For this review, take the finished solid that the model builds, in its own axes (mm). A direction names the side the tool comes from. Coordinates: 2 decimals unless noted, no trailing zeros. Order: outer loops, then holes, each group sorted by start corner. A loop starts at its lowest first (then second) coordinate and runs counter-clockwise, first axis right, second up. Notation, with made-up numbers: M 0.5,78 L 54.5,78 A20 ccw 54.5,115 Z; hole C 39.25,-29.5 d8. An arc over 180 degrees is marked long. Use one line per item in the form item = value. Start each with the question number.
```python
from build123d import *

# Parameters (mm, degrees)
SKETCH_1_R               = 5.65
SKETCH_1_R_2             = 4.15
EXTRUDE_1_DEPTH          = 8
SKETCH_1_3_R             = 11
SKETCH_1_3_R_2           = 5.65
EXTRUDE_2_DEPTH          = 4.75
CUT_EXTRUDE_1_DEPTH      = 3.5
CUT_EXTRUDE_START        = -3.25
CUT_EXTRUDE_3_DEPTH      = 3.25
CUT_EXTRUDE_START_2      = -10
CUT_EXTRUDE_4_DEPTH      = 10
PATTERN_CIRCULAR_1_COUNT = 35


with BuildPart() as part:
    # 草图1 → 凸台-拉伸1 (new body)
    with BuildSketch(Plane(origin=(0, 0, 0), x_dir=(1, 0, 0), z_dir=(0, 1, 0))):
        with Locations(Location((0, 0, 0), (0, 0, 270))):
            Circle(SKETCH_1_R)
        with Locations(Location((0, 0, 0), (0, 0, 270))):
            Circle(SKETCH_1_R_2, mode=Mode.SUBTRACT)
    extrude(amount=EXTRUDE_1_DEPTH)

    # 草图1<3> → 凸台-拉伸2 (add)
    with BuildSketch(Plane(origin=(0, 0, 0), x_dir=(1, 0, 0), z_dir=(0, 1, 0))):
        with Locations(Location((0, 0, 0), (0, 0, 270))):
            Circle(SKETCH_1_3_R)
        with Locations(Location((0, 0, 0), (0, 0, 270))):
            Circle(SKETCH_1_3_R_2, mode=Mode.SUBTRACT)
    extrude(amount=EXTRUDE_2_DEPTH)

    # 草图2 → 切除-拉伸1 (cut)
    with BuildSketch(Plane.XZ):
        Polygon((0, -7.274613392), (-6.3, -3.637306696), (-6.3, 3.637306696), (0, 7.274613392), (6.3, 3.637306696), (6.3, -3.637306696), align=None)
    extrude(amount=-CUT_EXTRUDE_1_DEPTH, mode=Mode.SUBTRACT)

    # 草图4 → 切除-拉伸3 (cut)
    with BuildSketch(Plane(origin=(0, 8, 0), x_dir=(1, 0, 0), z_dir=(0, 1, 0)).offset(CUT_EXTRUDE_START)):
        with BuildLine():
            Line((-2.1, 5.245235934), (-2.1, 3.579455266))
            ThreePointArc((-2.1, 3.579455266), (0, 4.15), (2.1, 3.579455266))
            Line((2.1, 3.579455266), (2.1, 5.245235934))
            ThreePointArc((2.1, 5.245235934), (0, 5.65), (-2.1, 5.245235934))
        make_face()
        with BuildLine():
            Line((2, -3.636275567), (2, -5.284174486))
            ThreePointArc((2, -5.284174486), (0, -5.65), (-2, -5.284174486))
            Line((-2, -5.284174486), (-2, -3.636275567))
            ThreePointArc((-2, -3.636275567), (0, -4.15), (2, -3.636275567))
        make_face()
    extrude(amount=CUT_EXTRUDE_3_DEPTH, mode=Mode.SUBTRACT)

    # 草图5 → 切除-拉伸4 (cut)
    with BuildSketch(Plane(origin=(0, 4.75, 0), x_dir=(1, 0, 0), z_dir=(0, 1, 0)).offset(CUT_EXTRUDE_START_2)):
        with BuildLine():
            ThreePointArc((0.574025149, 10.985012295), (0, 11), (-0.574025149, 10.985012295))
            Line((-0.574025149, 10.985012295), (-0.287012574, 10.292102646))
            Line((-0.287012574, 10.292102646), (0.287012574, 10.292102646))
            Line((0.287012574, 10.292102646), (0.574025149, 10.985012295))
        make_face()
    cut_extrude_4 = extrude(amount=CUT_EXTRUDE_4_DEPTH, mode=Mode.SUBTRACT)

    # 阵列(圆周)1: 切除-拉伸4 ×35 about axis
    pattern_circular_1_axis = Axis((0, 0, 0), (0, 1, 0))
    for i in range(1, PATTERN_CIRCULAR_1_COUNT):
        add(cut_extrude_4.rotate(pattern_circular_1_axis, i * 360 / PATTERN_CIRCULAR_1_COUNT), mode=Mode.SUBTRACT)


solid = part.part
```
1. Tool access review of faces 1 (the cylindrical face through (-5.65, 6.35, -0.04)), 2 (the flat face through (-6.3, 2, 0)), 3 (the flat face through (-2.1, 6, -4)), 4 (the flat face through (2, 6, 4)): name each direction out of +Z, -Z, +X, -X, +Y, -Y from which nothing blocks a thin tool from reaching the whole face with its end or side.
2. Consider section A-A, the plane y = 6.75. Write out the cut boundary in (x, z), plus the area to 3 significant figures.
3. To check wall thickness, follow line 1 (Z direction, x = 0, y = 4.6); line 2 (X direction, y = 5.25, z = 0); line 3 (X direction, y = 2.75, z = 1). State the ranges of each line that lie inside material, in increasing order.
4. For pin 1 Ø3 at (y, z) = (3.5, -5) entering from -X; pin 2 Ø0.8 at (y, z) = (7, -4) entering from -X; pin 3 Ø1.8 at (y, z) = (6.5, 5) entering from -X, all flat-tipped, find the tip position at first contact; note any pin that passes through.
5. The part is to be moulded in two halves that separate along Z. For faces 5 (the flat face through (4.3, 8, -0.1)), 6 (the flat face through (3.194, 1.726, -5.43)), 7 (the cylindrical face through (-10.723, 2.342, -2.453)), say which applies: pulls with the +Z half, pulls with the -Z half, needs draft (parallel to the pull), parting line crosses it, or undercut.
Answers follow:
q1.face_1 = -X, +Y
q1.face_2 = -Y
q1.face_3 = -Z, +Y
q1.face_4 = +Z, -Z, +Y
q2.outline = M -2.1,-5.25 L -2.1,-3.58 A4.15 cw -2,3.64 L -2,5.28 A5.65 ccw Z; M 2,3.64 A4.15 cw 2.1,-3.58 L 2.1,-5.25 A5.65 ccw 2,5.28 Z
q2.area = 33.5 mm²
q3.line_1 = -10.29 to -4.15, 4.15 to 11
q3.line_2 = -5.65 to -4.15, 4.15 to 5.65
q3.line_3 = -10.81 to -6.3, 6.3 to 10.81
q4.pin_1 = -10.27
q4.pin_2 = -4.35
q4.pin_3 = -3.89
q5.face_5 = needs draft
q5.face_6 = undercut
q5.face_7 = pulls with the -Z half
